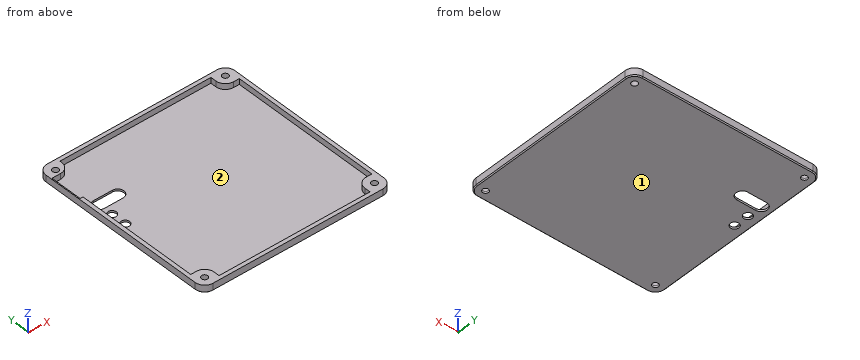
```python
from build123d import *

# Parameters (mm, degrees)
SKETCH_W        = 100
SKETCH_H        = 100
PAD_DEPTH       = 1
SKETCH001_W     = 100
SKETCH001_H     = 100
PAD001_DEPTH    = 3
SKETCH002_R     = 1.6
POCKET_DEPTH    = 3
FILLET_R        = 5
SKETCH004_R     = 2.25
POCKET001_DEPTH = 5
CHAMFER_SIZE    = 0.5


with BuildPart() as part:
    # Sketch → Pad (new body)
    with BuildSketch(Plane.XY):
        with Locations((50, 50)):
            Rectangle(SKETCH_W, SKETCH_H)
    extrude(amount=-PAD_DEPTH)

    # Sketch001 → Pad001 (join)
    with BuildSketch(Plane.XY):
        with Locations((50, 50)):
            Rectangle(SKETCH001_W, SKETCH001_H)
        Polygon((10, 10), (10, 2), (90, 2), (90, 10), (98, 10), (98, 90), (90, 90), (90, 98), (10, 98), (10, 92), (0.5, 92), (0.5, 75), (2, 75), (2, 10), align=None, mode=Mode.SUBTRACT)
    extrude(amount=PAD001_DEPTH)

    # Sketch002 → Pocket (cut, symmetric)
    with BuildSketch(Plane.XY):
        with Locations((5, 95)):
            Circle(SKETCH002_R)
        with Locations((5, 5)):
            Circle(SKETCH002_R)
        with Locations((95, 5)):
            Circle(SKETCH002_R)
        with Locations((95, 95)):
            Circle(SKETCH002_R)
    extrude(amount=POCKET_DEPTH, both=True, mode=Mode.SUBTRACT)

    # Fillet
    fillet_edges = [part.edges().sort_by_distance(p)[0] for p in [
        (100, 100, 1.5),
        (100, 0, 1.5),
        (0, 0, 1.5),
        (0, 100, 1.5),
        (10, 92, 1.5),
        (10, 10, 1.5),
        (90, 10, 1.5),
        (90, 90, 1.5),
    ]]
    fillet(fillet_edges, radius=FILLET_R)

    # Sketch004 (on DatumPlane) → Pocket001 (cut)
    with BuildSketch(Plane.XY):
        with Locations((6, 62)):
            Circle(SKETCH004_R)
        with Locations((6, 54)):
            Circle(SKETCH004_R)
        with BuildLine():
            ThreePointArc((6, 73.25), (2.75, 70), (6, 66.75))
            Line((6, 66.75), (16, 66.75))
            ThreePointArc((16, 66.75), (19.25, 70), (16, 73.25))
            Line((6, 73.25), (16, 73.25))
        make_face()
    extrude(amount=-POCKET001_DEPTH, mode=Mode.SUBTRACT)

    # Chamfer
    chamfer_edges = [part.edges().sort_by_distance(p)[0] for p in [
        (50, 0, -1),
    ]]
    chamfer(chamfer_edges, length=CHAMFER_SIZE)


solid = part.part
```
For this review, take the finished solid that the model builds, in its own axes (mm). Face numbers are marked on the shaded views. Round coordinates to 2 decimals unless told otherwise and drop trailing zeros. Order: outer loops, then holes, each group sorted by start corner. A loop starts at its lowest first (then second) coordinate and runs counter-clockwise, first axis right, second up. Notation, with made-up numbers: (-18.5, 5.5) -> (1.5, 5.5) arc R14 ccw to (1.5, 16.5) -> close; hole circle Ø4 at (-23, 29). An arc over 180 degrees is marked (long way). Use a Markdown table: item, result.
Item 1: Draft analysis for pull direction Y (two halves, no side actions). For the marked faces 1 and 2, state which applies: +Y half, -Y half, draft (parallel to the pull), parting line (faces both ways), or undercut.
Resolved:
| item | result |
|---|---|
| face 1 | draft |
| face 2 | undercut |
Item 2: Take a section at B-B (z = 1.4). State how many separate pieces and enclosed holes the cut face has, plus the area to 3 significant figures.
Resolved:
| item | result |
|---|---|
| separate pieces | 1 |
| enclosed holes | 5 |
| area | 923 mm² |
Item 3: Take a section at A-A (y = 54). State the section outline as (x, z) points.
Resolved:
| item | result |
|---|---|
| outline | (0, -0.5) -> (0.5, -1) -> (3.75, -1) -> (3.75, 0) -> (2, 0) -> (2, 3) -> (0, 3) -> close; (8.25, -1) -> (99.5, -1) -> (100, -0.5) -> (100, 3) -> (98, 3) -> (98, 0) -> (8.25, 0) -> close |
Item 4: For line 1 along Y through (x, z) = (95, 0.2); line 2 along X through (y, z) = (65, 0.8), list the stretches that pass through material, from the lowest coordinate up. Write a range as [from, to].
Resolved:
| item | result |
|---|---|
| line 1 | y = [0, 3.4], [6.6, 10], [90, 93.4], [96.6, 100] |
| line 2 | x = [0, 2], [98, 100] |
Item 5: Take a section at C-C (x = 43). State the section outline as (y, z) points.
Resolved:
| item | result |
|---|---|
| outline | (0, -0.5) -> (0.5, -1) -> (99.5, -1) -> (100, -0.5) -> (100, 3) -> (98, 3) -> (98, 0) -> (2, 0) -> (2, 3) -> (0, 3) -> close |
Item 6: For pin 1 (0.9 mm diameter, centred on x = 96.5, z = 1.5, fed in from -Y); pin 2 (10 mm diameter, centred on x = 23, y = 38, fed in from +Z), all flat-tipped, find the tip position at first contact; note any pin that passes through.
Resolved:
| item | result |
|---|---|
| pin 1 | stops at y = 0.11 |
| pin 2 | stops at z = 0 |
